Design review of the part built by this model. Coordinates are the model's own, in mm. Coordinates: 2 decimals unless noted, no trailing zeros. Loops run counter-clockwise (first coordinate to the right, second up) from the corner with the lowest first, then second, coordinate; pieces in that order, holes last. Notation, with made-up numbers: (-40, -14.75) -> (13, -14.75) arc R23 cw to (13, 17.25) -> close; hole circle Ø4 at (-30, 48). An arc over 180 degrees is marked (long way). Answer in a Markdown table with one row per item.
```python
from build123d import *

# Parameters (mm, degrees)
BOSS_EXTRUDE1_DEPTH                  = 165.66388
F_10_32_TAPPED_HOLE1_D               = 4.0386
F_10_32_TAPPED_HOLE1_DEPTH           = 16.34744
F_10_32_TAPPED_HOLE1_TIP             = 1.213317848
F_10_32_TAPPED_HOLE1_ON_FACE_2_D     = 4.0386
F_10_32_TAPPED_HOLE1_ON_FACE_2_DEPTH = 16.34744
F_10_32_TAPPED_HOLE1_ON_FACE_2_TIP   = 1.213317848


with BuildPart() as part:
    # Sketch1 → Boss-Extrude1 (new, symmetric)
    with BuildSketch(Plane.XY):
        with BuildLine():
            ThreePointArc((0.93173274, 6.79441227), (0, 6.858), (-0.93173274, 6.79441227))
            Line((-0.93173274, 6.79441227), (-5.41826726, 4.204110358))
            ThreePointArc((-5.41826726, 4.204110358), (-5.939202219, 3.429), (-6.35, 2.590301913))
            Line((-6.35, 2.590301913), (-6.35, -2.590301913))
            ThreePointArc((-6.35, -2.590301913), (-5.939202219, -3.429), (-5.41826726, -4.204110358))
            Line((-5.41826726, -4.204110358), (-0.93173274, -6.79441227))
            ThreePointArc((-0.93173274, -6.79441227), (0, -6.858), (0.93173274, -6.79441227))
            Line((0.93173274, -6.79441227), (5.41826726, -4.204110358))
            ThreePointArc((5.41826726, -4.204110358), (5.939202219, -3.429), (6.35, -2.590301913))
            Line((6.35, -2.590301913), (6.35, 2.590301913))
            ThreePointArc((6.35, 2.590301913), (5.939202219, 3.429), (5.41826726, 4.204110358))
            Line((5.41826726, 4.204110358), (0.93173274, 6.79441227))
        make_face()
    extrude(amount=BOSS_EXTRUDE1_DEPTH, both=True)

    # #10-32 Tapped Hole1
    with Locations(Plane.XY.offset(165.66388)):
        with Locations((0, 0)):
            Hole(F_10_32_TAPPED_HOLE1_D / 2, depth=F_10_32_TAPPED_HOLE1_DEPTH)
            with Locations((0, 0, -(F_10_32_TAPPED_HOLE1_DEPTH + F_10_32_TAPPED_HOLE1_TIP / 2))):  # 118° drill point
                Cone(0, F_10_32_TAPPED_HOLE1_D / 2, F_10_32_TAPPED_HOLE1_TIP, mode=Mode.SUBTRACT)

    # #10-32 Tapped Hole1 on face 2
    with Locations(Plane(origin=(0, 0, -165.66388), x_dir=(-1, 0, 0), z_dir=(0, 0, -1))):
        with Locations((0, 0)):
            Hole(F_10_32_TAPPED_HOLE1_ON_FACE_2_D / 2, depth=F_10_32_TAPPED_HOLE1_ON_FACE_2_DEPTH)
            with Locations((0, 0, -(F_10_32_TAPPED_HOLE1_ON_FACE_2_DEPTH + F_10_32_TAPPED_HOLE1_ON_FACE_2_TIP / 2))):  # 118° drill point
                Cone(0, F_10_32_TAPPED_HOLE1_ON_FACE_2_D / 2, F_10_32_TAPPED_HOLE1_ON_FACE_2_TIP, mode=Mode.SUBTRACT)


solid = part.part
```
(1) Take a section at A-A on z = 39. Give the boundary of the cut face in (x, y), and give its area (3 significant figures).
Evaluation:
| item | result |
|---|---|
| outline | (-6.35, -2.59) arc R6.86 ccw to (-5.42, -4.2) -> (-0.93, -6.79) arc R6.86 ccw to (0.93, -6.79) -> (5.42, -4.2) arc R6.86 ccw to (6.35, -2.59) -> (6.35, 2.59) arc R6.86 ccw to (5.42, 4.2) -> (0.93, 6.79) arc R6.86 ccw to (-0.93, 6.79) -> (-5.42, 4.2) arc R6.86 ccw to (-6.35, 2.59) -> close |
| area | 137 mm² |
(2) For pin 1 (5.5 mm diameter, centred on x = 0, y = 0, fed in from +Z); pin 2 (3.5 mm diameter, centred on x = 0, y = 0, fed in from +Z); pin 3 (1.5 mm diameter, centred on x = 2, z = 113.5, fed in from -Y); pin 4 (4 mm diameter, centred on x = 5, z = -131.5, fed in from -Y), all flat-tipped, find the tip position at first contact; note any pin that passes through.
Evaluation:
| item | result |
|---|---|
| pin 1 | stops at z = 165.66 |
| pin 2 | stops at z = 149.15 |
| pin 3 | stops at y = -6.61 |
| pin 4 | stops at y = -5.6 |
(3) To check wall thickness, follow probe 1 along X at (y, z) = (0, -155.5); probe 2 along Y at (x, z) = (0, 161.75); probe 3 along Y at (x, z) = (-0.75, 23.5). State the ranges of each line that lie inside material, in increasing order.
Evaluation:
| item | result |
|---|---|
| probe 1 | x = -6.35 to -2.02, 2.02 to 6.35 |
| probe 2 | y = -6.86 to -2.02, 2.02 to 6.86 |
| probe 3 | y = -6.82 to 6.82 |
